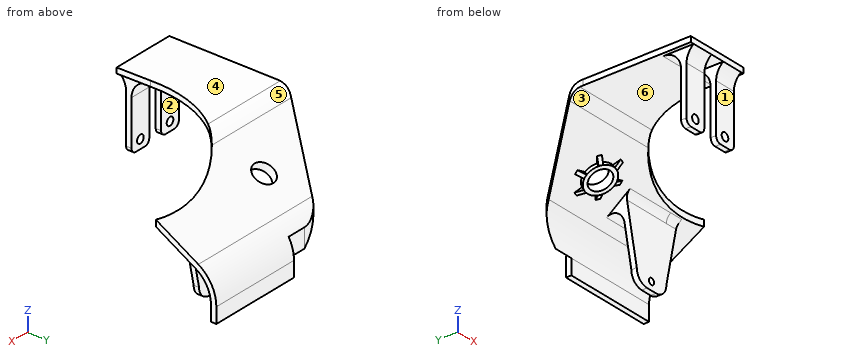
```python
from build123d import *

# Parameters (mm, degrees)
SALIENTE_EXTRUIR1_DEPTH  = 58.05
REDONDEO1_R              = 20
REDONDEO2_R              = 20
REDONDEO3_R              = 17
REDONDEO4_R              = 17
CAVIDAD1_START           = -47
CAVIDAD1_DEPTH           = 51
CROQUIS8_W               = 12
CROQUIS8_H               = 3
SALIENTE_EXTRUIR2_DEPTH  = 38
CROQUIS9_R               = 2.25
CORTAR_EXTRUIR6_DEPTH    = 135.588949923
SALIENTE_EXTRUIR3_REACH  = 146.947
CROQUIS11_W              = 20
CROQUIS11_H              = 3
CROQUIS12_W              = 69.238292886
CROQUIS12_H              = 3
CORTAR_EXTRUIR7_DEPTH    = 1
CROQUIS15_R              = 1.75
CORTAR_EXTRUIR10_DEPTH   = 5
REDONDEO5_R              = 7
REDONDEO6_R              = 3
CROQUIS18_R              = 6
CORTAR_EXTRUIR12_DEPTH   = 146.081609054
CROQUIS19_R              = 8.25
CROQUIS19_R_2            = 6
SALIENTE_EXTRUIR4_DEPTH  = 2
CROQUIS16_R              = 65
CORTAR_EXTRUIR11_DEPTH   = 145.946782753
SALIENTE_EXTRUIR5_DEPTH  = 3
NERVIO8_START            = -1.125
NERVIO8_DEPTH            = 2.25
MATRIZC2_COUNT           = 6
REDONDEO6_OF_SIMETR_A1_R = 3
REDONDEO7_R              = 10
REDONDEO8_R              = 10
REDONDEO9_R              = 6
CORTAR_EXTRUIR14_DEPTH   = 145.946782753
REDONDEO10_R             = 5


with BuildPart() as part:
    # Croquis1 → Saliente-Extruir1 (new, symmetric)
    with BuildSketch(Plane(origin=(0, 0, 0), x_dir=(0, 0, -1), z_dir=(1, 0, 0))):
        Polygon((0, 0), (0, 67.196152423), (28.732050808, 116.961524227), (47, 116.961524227), (47, 119.961524227), (27, 119.961524227), (-3, 68), (-3, 0), align=None)
    extrude(amount=SALIENTE_EXTRUIR1_DEPTH, both=True)

    # Redondeo1
    redondeo1_edges = [part.edges().sort_by_distance(p)[0] for p in [
        (0, 68, 3),
    ]]
    fillet(redondeo1_edges, radius=REDONDEO1_R)

    # Redondeo2
    redondeo2_edges = [part.edges().sort_by_distance(p)[0] for p in [
        (0, 119.961524227, -27),
    ]]
    fillet(redondeo2_edges, radius=REDONDEO2_R)

    # Redondeo3
    redondeo3_edges = [part.edges().sort_by_distance(p)[0] for p in [
        (0, 116.961524227, -28.732050808),
    ]]
    fillet(redondeo3_edges, radius=REDONDEO3_R)

    # Redondeo4
    redondeo4_edges = [part.edges().sort_by_distance(p)[0] for p in [
        (0, 67.196152423, 0),
    ]]
    fillet(redondeo4_edges, radius=REDONDEO4_R)

    # Cavidad1: read off the stored shape, not the designer's step
    # Cavidad1 outline → Cavidad1 (cut)
    with BuildSketch(Plane.XY.offset(CAVIDAD1_START)):
        with BuildLine():
            Line((58.05, 0), (58.05, 119.961524227))
            Line((58.05, 119.961524227), (-5.55, 119.961524227))
            Line((-5.55, 119.961524227), (-5.55, 116.961524227))
            Line((-5.55, 116.961524227), (5.123846837, 116.961524227))
            ThreePointArc((5.123846837, 116.961524227), (12.308357287, 115.368756607), (18.14660237, 110.888913592))
            Line((18.14660237, 110.888913592), (51.073651347, 71.647984679))
            ThreePointArc((51.073651347, 71.647984679), (54.025670368, 66.534937751), (55.050895814, 60.720595315))
            Line((55.050895814, 60.720595315), (55.050895814, 0))
            Line((55.050895814, 0), (58.05, 0))
        make_face()
    extrude(amount=CAVIDAD1_DEPTH, mode=Mode.SUBTRACT)

    # Croquis8 → Saliente-Extruir2 (add)
    with BuildSketch(Plane(origin=(0, 0, 0), x_dir=(-1, 0, 0), z_dir=(0, 0, -1))):
        with Locations((-47.050895814, 6.5)):
            Rectangle(CROQUIS8_W, CROQUIS8_H)
    saliente_extruir2 = extrude(amount=SALIENTE_EXTRUIR2_DEPTH)

    # Croquis9 → Cortar-Extruir6 (cut, through all)
    with BuildSketch(Plane(origin=(0, 8, 0), x_dir=(1, 0, 0), z_dir=(0, 1, 0))):
        with Locations(Location((47.050895814, 33, 0), (0, 0, 180))):
            Circle(CROQUIS9_R)
    cortar_extruir6 = extrude(amount=-CORTAR_EXTRUIR6_DEPTH, mode=Mode.SUBTRACT)

    # Saliente-Extruir3: up to this plane
    saliente_extruir3_end = Plane(origin=(58.05, 67.196152423, 0), z_dir=(0, 0.49999999999999767, 0.86602540378444))
    # Croquis11 → Saliente-Extruir3 (add, up to the surface)
    with BuildSketch(Plane(origin=(0, 0, -54), x_dir=(-1, 0, 0), z_dir=(0, 0, -1)), mode=Mode.PRIVATE) as saliente_extruir3_sk1:
        with Locations((28.05, 92.461524227)):
            Rectangle(CROQUIS11_W, CROQUIS11_H)
    saliente_extruir3_tool1 = split(extrude(saliente_extruir3_sk1.sketch, amount=-SALIENTE_EXTRUIR3_REACH, mode=Mode.PRIVATE), bisect_by=saliente_extruir3_end, keep=Keep.BOTH, mode=Mode.PRIVATE)
    add(saliente_extruir3_tool1.solids().sort_by_distance((-28.05, 92.461524, -54))[0])

    # Croquis12 → Cortar-Extruir7 (cut)
    with BuildSketch(Plane.XZ):
        with Locations((20.431749371, 1.5)):
            Rectangle(CROQUIS12_W, CROQUIS12_H)
    extrude(amount=-CORTAR_EXTRUIR7_DEPTH, mode=Mode.SUBTRACT)

    # Croquis15 → Cortar-Extruir10 (cut)
    with BuildSketch(Plane.XZ.offset(-90.961524227)):
        with Locations(Location((-28.049104186, -49.5, 0), (0, 0, 270))):
            Circle(CROQUIS15_R)
    extrude(amount=-CORTAR_EXTRUIR10_DEPTH, mode=Mode.SUBTRACT)

    # Redondeo5
    redondeo5_edges = [part.edges().sort_by_distance(p)[0] for p in [
        (-18.05, 92.461524227, -54),
        (-38.05, 92.461524227, -54),
    ]]
    fillet(redondeo5_edges, radius=REDONDEO5_R)

    # Redondeo6
    redondeo6_edges = [part.edges().sort_by_distance(p)[0] for p in [
        (53.050895814, 6.5, -38),
        (41.050895814, 6.5, -38),
    ]]
    fillet(redondeo6_edges, radius=REDONDEO6_R)

    # Croquis18 → Cortar-Extruir12 (cut, through all)
    with BuildSketch(Plane(origin=(0, 18.299038106, 31.694863729), x_dir=(1, 0, 0), z_dir=(0, 0.4999999999999976, 0.86602540378444))):
        with Locations(Location((7.567578046, 85.748711306, 0), (0, 0, 270))):
            Circle(CROQUIS18_R)
    extrude(amount=-CORTAR_EXTRUIR12_DEPTH, mode=Mode.SUBTRACT)

    # Croquis19 → Saliente-Extruir4 (add)
    with BuildSketch(Plane(origin=(0, 16.799038106, 29.096787517), x_dir=(-1, 0, 0), z_dir=(0, -0.4999999999999977, -0.8660254037844399))):
        with Locations(Location((-7.567578046, 85.748711306, 0), (0, 0, 270))):
            Circle(CROQUIS19_R)
        with Locations(Location((-7.567578046, 85.748711306, 0), (0, 0, 270))):
            Circle(CROQUIS19_R_2, mode=Mode.SUBTRACT)
    extrude(amount=SALIENTE_EXTRUIR4_DEPTH)

    # Croquis16 → Cortar-Extruir11 (cut, through all)
    with BuildSketch(Plane.XY.offset(3)):
        with Locations((-45.071920691, 22.721524227)):
            Circle(CROQUIS16_R)
    extrude(amount=-CORTAR_EXTRUIR11_DEPTH, mode=Mode.SUBTRACT)

    # Croquis25 → Saliente-Extruir5 (add)
    with BuildSketch(Plane.XZ.offset(-90.961524227)):
        Polygon((-38.05, -13.720943809), (-45.254421175, -13.720943809), (-38.05, -47), align=None)
        Polygon((-10.845578825, -13.720943809), (-18.05, -47), (-18.05, -13.720943809), align=None)
    extrude(amount=-SALIENTE_EXTRUIR5_DEPTH)

    # Nervio8: read off the stored shape, not the designer's step
    # Nervio8 outline → Nervio8 (add)
    with BuildSketch(Plane(origin=(46.658144676, 40.407138583, -23.329072338), x_dir=(-0.7071067811865435, 0.6123724356957997, -0.353553390593273), z_dir=(-0.7071067811865517, -0.612372435695792, 0.35355339059327007)).offset(NERVIO8_START)):
        Polygon((47.10947397, -31.598076211), (47.032409489, -31.598076211), (43.032409489, -33.598076211), (47.10947397, -33.598076211), align=None)
    nervio8 = extrude(amount=NERVIO8_DEPTH)

    # MatrizC2: Nervio8 ×6 about axis
    matrizc2_axis = Axis((7.567578046, 74.260562333, -42.874355653), (0, -0.49999999999999767, -0.86602540378444))
    for i in range(1, MATRIZC2_COUNT):
        add(nervio8.rotate(matrizc2_axis, i * 360 / MATRIZC2_COUNT))

    # Simetría1: Saliente-Extruir2, Cortar-Extruir6 across plane
    add(saliente_extruir2.mirror(Plane(origin=(37.050895814, 0, 0), x_dir=(0, 0, 1), z_dir=(1, 0, 0))))
    add(cortar_extruir6.mirror(Plane(origin=(37.050895814, 0, 0), x_dir=(0, 0, 1), z_dir=(1, 0, 0))), mode=Mode.SUBTRACT)

    # Redondeo6 of Simetría1
    redondeo6_of_simetr_a1_edges = [part.edges().sort_by_distance(p)[0] for p in [
        (21.050895814, 6.5, -38),
        (33.050895814, 6.5, -38),
    ]]
    fillet(redondeo6_of_simetr_a1_edges, radius=REDONDEO6_OF_SIMETR_A1_R)

    # Redondeo7
    # the kernel refuses this fillet: 10 mm, written as the material it adds along each edge
    with BuildSketch(Plane(origin=(21.050895814, 5, 0), x_dir=(0, -1, 0), z_dir=(1, 0, 0))) as redondeo7_piece_1_section:
        with BuildLine():
            CenterArc((10, 8), REDONDEO7_R, 180, 53.130102354)
            Line((0, 8), (-0.2, 8))
            Line((-0.2, 8), (-0.2, 0))
            Line((-0.2, 0), (0, -0.2))
            ThreePointArc((0, -0.2), (2, -0.2), (3.88, -0.16))
            Line((3.88, -0.16), (4, 0))
        make_face()
    redondeo7_piece_1 = extrude(amount=32, mode=Mode.PRIVATE)
    redondeo7_piece_1 = split(redondeo7_piece_1, bisect_by=Plane(origin=(33.050895814, 5, 0), z_dir=(-1, 0, 0)), keep=Keep.TOP, mode=Mode.PRIVATE)
    add(redondeo7_piece_1)
    with BuildSketch(Plane(origin=(41.050895814, 5, 0), x_dir=(0, -1, 0), z_dir=(1, 0, 0))) as redondeo7_piece_2:
        with BuildLine():
            CenterArc((10, 8), REDONDEO7_R, 180, 53.130102354)
            Line((0, 8), (-0.2, 8))
            Line((-0.2, 8), (-0.2, 0))
            Line((-0.2, 0), (0, -0.2))
            ThreePointArc((0, -0.2), (2, -0.2), (3.88, -0.16))
            Line((3.88, -0.16), (4, 0))
        make_face()
    extrude(amount=12)
    with BuildSketch(Plane(origin=(53.050895814, 5, 0), x_dir=(0, -1, 0), z_dir=(-1, 0, 0))) as redondeo7_piece_3_section:
        with BuildLine():
            CenterArc((10, -8), REDONDEO7_R, 126.869897646, 53.130102354)
            Line((0, -8), (-0.2, -8))
            Line((-0.2, -8), (-0.2, 0))
            Line((-0.2, 0), (0, 0.2))
            ThreePointArc((0, 0.2), (2, 0.2), (3.88, 0.16))
            Line((3.88, 0.16), (4, 0))
        make_face()
    redondeo7_piece_3 = extrude(amount=32, mode=Mode.PRIVATE)
    redondeo7_piece_3 = split(redondeo7_piece_3, bisect_by=Plane(origin=(41.050895814, 5, 0), z_dir=(1, 0, 0)), keep=Keep.TOP, mode=Mode.PRIVATE)
    add(redondeo7_piece_3)
    with BuildSketch(Plane(origin=(33.050895814, 5, 0), x_dir=(0, -1, 0), z_dir=(-1, 0, 0))) as redondeo7_piece_4:
        with BuildLine():
            CenterArc((10, -8), REDONDEO7_R, 126.869897646, 53.130102354)
            Line((0, -8), (-0.2, -8))
            Line((-0.2, -8), (-0.2, 0))
            Line((-0.2, 0), (0, 0.2))
            ThreePointArc((0, 0.2), (2, 0.2), (3.88, 0.16))
            Line((3.88, 0.16), (4, 0))
        make_face()
    extrude(amount=12)

    # Redondeo8
    redondeo8_edges = [part.edges().sort_by_distance(p)[0] for p in [
        (47.050895814, 8, 0),
        (27.050895814, 8, 0),
    ]]
    fillet(redondeo8_edges, radius=REDONDEO8_R)

    # Redondeo9
    redondeo9_edges = [part.edges().sort_by_distance(p)[0] for p in [
        (-28.05, 93.961524227, -15.452994616),
    ]]
    fillet(redondeo9_edges, radius=REDONDEO9_R)

    # Croquis31 → Cortar-Extruir14 (cut, through all)
    with BuildSketch(Plane.XY.offset(3)):
        with BuildLine():
            Line((16.191244305, 1), (19.497703143, 1))
            Line((19.497703143, 1), (19.844268253, 19.421764692))
            ThreePointArc((19.844268253, 19.421764692), (18.686590065, 10.078253042), (16.191244305, 1))
        make_face()
    extrude(amount=-CORTAR_EXTRUIR14_DEPTH, mode=Mode.SUBTRACT)

    # Redondeo10
    redondeo10_edges = [part.edges().sort_by_distance(p)[0] for p in [
        (-28.05, 90.961524227, -13.720943809),
    ]]
    fillet(redondeo10_edges, radius=REDONDEO10_R)


with BuildPart() as body_2:
    # Simetría2: mirrored copy
    add(part.part.mirror(Plane(origin=(-58.05, 0, 0), x_dir=(0, 0, 1), z_dir=(1, 0, 0))))


solid = body_2.part
```
The listing builds one solid part. Answer for the finished solid, in the listing's coordinates (mm). Face numbers are marked on the shaded views. A direction names the side the tool comes from. Give positions to 0.01 mm unless a question says otherwise; leave off trailing zeros. Loops run counter-clockwise (first coordinate to the right, second up) from the corner with the lowest first, then second, coordinate; pieces in that order, holes last. Notation, with made-up numbers: (-28, -34) - (10, -34) arc R23 ccw to (10, 5) - close; hole circle Ø9 at (61.25, -37.5). An arc over 180 degrees is marked (long way). Return JSON: item names as keys, results as strings. Group by question number.
1. Which of the six approach directions +Z, -Z, +X, -X, +Y, -Y give full straight-line access (tool end or side, diameter ignored) to the marked faces 1, 2 and 3?
2. Given pin 1 Ø1.5 at (x, y) = (-155, 60) entering from -Z; pin 2 Ø5 at (y, z) = (7.5, -18.5) entering from -X; pin 3 Ø13.5 at (y, z) = (10, -24.5) entering from +X, each flat-ended and moving along its own axis, determine where each tip first touches the part or whether it passes through.
3. Find section B-B (z = -49.5). Write down the section's boundary in (x, y), then the cut area to 3 significant figures.
4. Find section D-D (z = -33). Write down the section's boundary in (x, y).
5. Find section A-A (z = -4). Write down the section's boundary in (x, y).
6. Determine the mould class of the marked faces 4, 5 and 6 for opening direction Y: pulls with the +Y half, pulls with the -Y half, needs draft (parallel to the pull), parting line crosses it, or undercut.
7. Straight lines are drawn through the part: line 1 (Z direction, x = -147, y = 43); line 2 (Y direction, x = -146, z = -12.5); line 3 (Y direction, x = -74, z = -45.5). For each, find the intervals that lie inside material, in ascending order. Write a range as [from, to].
8. Find section C-C (x = -67). Write down the section's boundary in (y, z), then the cut area to 3 significant figures.
Verdict:
{
 "1": {"face 1": "-Z, +X, -X, -Y", "face 2": "-Z, +X, -X, +Y", "face 3": "-Z, +X, -X"},
 "2": {"pin 1": "stops at z = 0", "pin 2": "stops at x = -169.15", "pin 3": "stops at x = -137.15"},
 "3": {"outline": "(-97.59, 90.96) - (-89.8, 90.96) - (-89.8, 93.96) - (-97.59, 93.96) - close; (-86.3, 90.96) - (-78.51, 90.96) - (-78.51, 93.96) - (-86.3, 93.96) - close", "area": "46.7 mm^2"},
 "4": {"outline": "(-169.15, 5) - (-165.4, 5) - (-165.4, 8) - (-169.15, 8) - close; (-160.9, 5) - (-157.15, 5) - (-157.15, 8) - (-160.9, 8) - close; (-149.15, 5) - (-145.4, 5) - (-145.4, 8) - (-149.15, 8) - close; (-140.9, 5) - (-137.15, 5) - (-137.15, 8) - (-140.9, 8) - close; (-126.77, 116.03) - (-58.05, 116.03) - (-58.05, 119.18) - (-110.55, 119.18) - (-110.55, 116.96) - (-121.22, 116.96) arc R17 ccw to start; (-101.08, 90.96) - (-75.02, 90.96) - (-75.02, 93.96) - (-101.08, 93.96) - close"},
 "5": {"outline": "(-169.15, 4.17) - (-157.15, 4.17) - (-157.15, 10) - (-169.15, 10) - close; (-165.1, 74.12) - (-110.81, 74.12) arc R65 cw to (-101.52, 80.12) - (-160.06, 80.12) - close; (-149.15, 4.17) - (-137.15, 4.17) - (-137.15, 10) - (-149.15, 10) - close"},
 "6": {"face 4": "needs draft", "face 5": "pulls with the +Y half", "face 6": "undercut"},
 "7": {"line 1": "z = [0, 3]", "line 2": "y = [5, 8], [88.85, 94.85]", "line 3": "y = [116.96, 119.96]"},
 "8": {"outline": "(87.6, -11.78) - (108.46, -23.82) arc R17 cw to (116.96, -38.55) - (116.96, -47) - (119.96, -47) - (119.96, -38.55) arc R20 ccw to (109.96, -21.23) - (87.6, -8.31) - close", "area": "158 mm^2"}
}
